Source: CAD feature listing. Evaluate the final solid. Frame: model axes, mm. A direction names the side the tool comes from. Round coordinates to 2 decimals unless told otherwise and drop trailing zeros. Order: outer loops, then holes, each group sorted by start corner. A loop starts at its lowest first (then second) coordinate and runs counter-clockwise, first axis right, second up. Notation, with made-up numbers: M 7.25,81.25 L 47.25,81.25 A15 cw 47.25,95.25 Z; hole C 34.25,0 d1. An arc over 180 degrees is marked long. Answer as CSV lines item,"result". Start each with the question number.
Item 1: First-contact query: P1, Ø6, axis at x = 67.5, y = -23.5, coming from the -Z side; P2, Ø5, axis at x = 10, z = 30.5, coming from the -Y side (3 decimals); P3, Ø10, axis at x = 70.5, y = 7, coming from the -Z side. Flat tips, straight axial feed; report the tip coordinate or a pass-through.
Item 2: Section query A-A on z = 5. Return the cut outline in (x, y).
Item 3: Section query B-B on y = 18. Return the cut outline in (x, z) (3 decimals).
Item 4: Section query C-C on x = 102. Return the cut outline in (y, z).
Item 5: Set-up query: faces 1 (the face through (47.7, -0.36, 40.25)), 2 (the face through (112.363, 9.728, 53.08)), 3 (the face through (42.64, 61.59, 0.13)), 4 (the face through (28.575, -18, 21)), 5 (the face through (36.8, 17.4, 51.8)). Return all of +Z, -Z, +X, -X, +Y, -Y with unobstructed straight access to the full face (end or side cutting, diameter ignored); none if empty.
Item 6: Pull-direction query (X, two-part tool) for faces 6 (the face through (36.8, -17.6, 51.8)), 7 (the face through (44.45, -1, 6)), 8 (the face through (61, 0, 43.683)); classes: +X half, -X half, draft (parallel to the pull), parting line (faces both ways), or undercut.
Item 7: Section query D-D on y = -40. Return the cut outline in (x, z) (3 decimals), plus the area to 3 significant figures.
Item 8: Line query: line 1 (Y direction, x = 62.5, z = 49); line 2 (Z direction, x = -25, y = -42) (3 decimals); line 3 (X direction, y = 10.5, z = 7). Output: solid intervals per line, ascending. Write a range as [from, to].
from build123d import *

# Parameters (mm, degrees)
F1_DEPTH = 63.5
F0_W     = 25.4
F0_H     = 15.875
F2_DEPTH = 25.4
F3_DEPTH = 9.525
F5_R     = 6.35


with BuildPart() as f1:
    # F0 (on Front) → F1 (new body, symmetric)
    with BuildSketch(Plane.XZ):
        Polygon((-44.45, -9.525), (44.45, -9.525), (44.45, 9.525), (28.575, 9.525), (-44.45, 9.525), align=None)
    extrude(amount=F1_DEPTH, both=True)

    # F0 (on Front) → F2 (join, symmetric)
    with BuildSketch(Plane.XZ):
        with BuildLine():
            Line((28.575, 9.525), (44.45, 9.525))
            Line((44.45, 9.525), (44.45, 32.2810681378))
            ThreePointArc((44.45, 32.2810681378), (47.7894660102, 40.3432522706), (55.851650143, 43.6827182808))
            Line((55.851650143, 43.6827182808), (63.5, 43.6827182808))
            Line((63.5, 43.6827182808), (63.5, 59.5577182808))
            Line((63.5, 59.5577182808), (55.851650143, 59.5577182808))
            ThreePointArc((55.851650143, 59.5577182808), (36.5641458588, 51.568572422), (28.575, 32.2810681378))
            Line((28.575, 32.2810681378), (28.575, 9.525))
        make_face()
        with Locations((76.2, 51.6202182808)):
            Rectangle(F0_W, F0_H)
    extrude(amount=F2_DEPTH, both=True)

    # F0 (on Front) → F3 (join, symmetric)
    with BuildSketch(Plane.XZ):
        with BuildLine():
            add(Edge.make_bspline(
                [(-44.45, 9.525), (-42.0993748289, 13.5310159807), (31.447590693, 8.169184866), (-11.7146146139, 63.4179972105), (63.5, 59.5577182808)],
                knots=[0, 0, 0, 0, 0.4393913897, 1, 1, 1, 1], degree=3))
            Line((-44.45, 9.525), (28.575, 9.525))
            Line((28.575, 9.525), (28.575, 32.2810681378))
            ThreePointArc((28.575, 32.2810681378), (36.5641458588, 51.568572422), (55.851650143, 59.5577182808))
            Line((55.851650143, 59.5577182808), (63.5, 59.5577182808))
        make_face()
    extrude(amount=F3_DEPTH, both=True)

    # F0 (on Front) → F4 (revolve)
    with BuildSketch(Plane.XZ):
        Polygon((88.9, 68.7322870837), (88.9, 59.5577182808), (88.9, 43.6827182808), (88.9, 36.9822870837), (114.3, 36.9822870837), (114.3, 68.7322870837), align=None)
    revolve(axis=Axis((88.9, 0, 52.8572870837), (0, 0, -1)))

    # F5
    f5_edges = [f1.edges().sort_by_distance(p)[0] for p in [
        (-44.45, -63.5, 0),
        (44.45, -63.5, 0),
        (44.45, 63.5, 0),
        (-44.45, 63.5, 0),
    ]]
    fillet(f5_edges, radius=F5_R)


solid = f1.part
Results:
1,P1,"z = 43.68"
1,P2,"y = -9.525"
1,P3,"z = 36.98"
2,outline,"M -44.45,-57.15 A6.35 ccw -38.1,-63.5 L 38.1,-63.5 A6.35 ccw 44.45,-57.15 L 44.45,57.15 A6.35 ccw 38.1,63.5 L -38.1,63.5 A6.35 ccw -44.45,57.15 Z"
3,outline,"M -44.45,-9.525 L 44.45,-9.525 L 44.45,32.281 A11.402 cw 55.852,43.683 L 70.979,43.683 L 70.979,36.982 L 106.821,36.982 L 106.821,68.732 L 70.979,68.732 L 70.979,59.558 L 55.852,59.558 A27.277 ccw 28.575,32.281 L 28.575,9.525 L -44.45,9.525 Z"
4,outline,"M -21.76,36.98 L 21.76,36.98 L 21.76,68.73 L -21.76,68.73 Z"
5,face 1,"-Z, +Y, -Y"
5,face 2,"none"
5,face 3,"+Z, -Z, +X, +Y"
5,face 4,"+Z, -X, -Y"
5,face 5,"+Z, -X, +Y"
6,face 6,"-X half"
6,face 7,"+X half"
6,face 8,"undercut"
7,outline,"M -44.45,-9.525 L 44.45,-9.525 L 44.45,9.525 L -44.45,9.525 Z"
7,area,"1,690 mm^2"
8,line 1,"[-25.4, 25.4]"
8,line 2,"[-9.525, 9.525]"
8,line 3,"[-44.45, 44.45]"
